Input: part model. Units: mm. Frame: model coordinates. A direction names the side the tool comes from. Round coordinates to 2 decimals unless told otherwise and drop trailing zeros. Loops run counter-clockwise (first coordinate to the right, second up) from the corner with the lowest first, then second, coordinate; pieces in that order, holes last.
(1) Access query for faces 4 (the face through (-4.289, -14.304, 1.972)), 5 (the face through (-6, -26, 2)), 6 (the face through (6, -12.5, 2)), 7 (the face through (-5, 0, 10)). Directions: +Z, -Z, +X, -X, +Y, -Y. A direction counts if a zero-diameter tool reaches every point of the face in a straight line with its end or side. Return the directions, or none.
(2) Cut plane A-A, the plane y = 0. Output: boundary loops of the cut face in (x, z) (3 decimals).
(3) Cut plane B-B, the plane x = -4.75. Output: boundary loops of the cut face in (y, z).
(4) First-contact query: pin 1 Ø12 at (x, z) = (-8.5, 47.5) entering from +Y; pin 2 Ø5 at (x, y) = (-1, 0) entering from -Z; pin 3 Ø1 at (y, z) = (5, 43) entering from -X; pin 4 Ø5 at (x, y) = (1.5, -18.5) entering from -Z. Flat tips, straight axial feed; report the tip coordinate or a pass-through.
(5) Cut plane D-D, the plane y = 18.5. Output: boundary loops of the cut face in (x, z), and give its area (3 significant figures).
(6) Draft query along Y for faces 1 (the face through (0, 8, 0)), 2 (the face through (5, -32.5, 33)), 3 (the face through (3, -23, 4)). Return one class per face: released by +Y, released by -Y, zero draft, split by the parting line, or undercut.
(7) Line query: line 1 (Y direction, x = 0, z = 5.6) (3 decimals); line 2 (Y direction, x = 0, z = 1.5) (3 decimals); line 3 (X direction, y = 9, z = 57.5). Output: solid intervals per line, ascending.
(8) Cut plane C-C, the plane z = 59.5. Output: boundary loops of the cut face in (x, y), and give its area (3 significant figures).
from build123d import *

# Parameters (mm, degrees)
F0_W     = 25
F0_H     = 65
F1_DEPTH = 10
F2_W     = 10
F2_H     = 65
F3_DEPTH = 57
F4_R     = 3.175
F5_DEPTH = 6
F7_DEPTH = 4
F8_R     = 3.175
F9_DEPTH = 3


with BuildPart() as f1:
    # F0 (on Top) → F1 (new body)
    with BuildSketch(Plane.XY):
        Rectangle(F0_W, F0_H)
    extrude(amount=F1_DEPTH)

    # F2 (on face) → F3 (join)
    with BuildSketch(Plane.XY.offset(10)):
        with Locations((7.5, 0)):
            Rectangle(F2_W, F2_H)
    extrude(amount=F3_DEPTH)

    # F4 (on face) → F5 (cut)
    with BuildSketch(Plane(origin=(0, 0, 0), x_dir=(1, 0, 0), z_dir=(0, 0, -1))):
        Circle(F4_R)
    extrude(amount=-F5_DEPTH, mode=Mode.SUBTRACT)

    # F6 (on face) → F7 (cut)
    with BuildSketch(Plane(origin=(0, 0, 0), x_dir=(1, 0, 0), z_dir=(0, 0, -1))):
        with BuildLine():
            Line((6, 24.5), (6, 52.5))
            Line((6, 52.5), (-6, 52.5))
            Line((-6, 52.5), (-6, 18.5))
            ThreePointArc((-6, 18.5), (-4.242641, 14.257359), (0, 12.5))
            ThreePointArc((0, 12.5), (4.242641, 14.257359), (6, 18.5))
            Line((6, 18.5), (6, 24.5))
        make_face()
        with BuildLine():
            Line((29.926794, 24.5), (6, 24.5))
            Line((6, 24.5), (6, 18.5))
            ThreePointArc((6, 18.5), (4.242641, 14.257359), (0, 12.5))
            Line((0, 12.5), (29.926794, 12.5))
            Line((29.926794, 12.5), (29.926794, 24.5))
        make_face()
    extrude(amount=-F7_DEPTH, mode=Mode.SUBTRACT)

    # F8 (on face) → F9 (cut)
    with BuildSketch(Plane(origin=(0, 0, 4), x_dir=(1, 0, 0), z_dir=(0, 0, -1))):
        with Locations((0, 18.5)):
            Circle(F8_R)
    extrude(amount=-F9_DEPTH, mode=Mode.SUBTRACT)


solid = f1.part
Reported:
1. face 4: -Z, +X, -Y
1. face 5: -Z, -Y
1. face 6: -Z, +X
1. face 7: +Z, -X, +Y, -Y
2. outline: (-12.5, 0) - (-3.175, 0) - (-3.175, 6) - (3.175, 6) - (3.175, 0) - (12.5, 0) - (12.5, 67) - (2.5, 67) - (2.5, 10) - (-12.5, 10) - close
3. outline: (-32.5, 4) - (-14.83, 4) - (-14.83, 0) - (32.5, 0) - (32.5, 10) - (-32.5, 10) - close
4. pin 1: passes through
4. pin 2: stops at z = 0
4. pin 3: stops at x = 2.5
4. pin 4: stops at z = 4
5. outline: (-12.5, 0) - (12.5, 0) - (12.5, 67) - (2.5, 67) - (2.5, 10) - (-12.5, 10) - close
5. area: 820 mm2
6. face 1: zero draft
6. face 2: released by -Y
6. face 3: undercut
7. line 1: y = -32.5 to -21.675, -15.325 to -3.175, 3.175 to 32.5
7. line 2: y = -12.5 to -3.175, 3.175 to 32.5
7. line 3: x = 2.5 to 12.5
8. outline: (2.5, -32.5) - (12.5, -32.5) - (12.5, 32.5) - (2.5, 32.5) - close
8. area: 650 mm2
